from build123d import *

# Parameters (mm, degrees)
FILLET1_R             = 0.2
HEX_START             = -1.9
HEX_2_DEPTH           = 1.9
THDSCHPAT_COUNT       = 10
THDSCHPAT_PITCH       = 0.73
BODY_MOVE_COPY1_ANGLE = 90


with BuildPart() as part:
    # BodySke → BaseBody (revolve)
    with BuildSketch(Plane.XY, mode=Mode.PRIVATE) as basebody_sk:
        Polygon((0, 0), (0, 4.875), (0.725, 4.875), (3.1, 2.5), (11.555, 2.5), (12, 2.055), (12, 0), align=None)
    revolve(basebody_sk.sketch.rotate(Axis((0, 0, 0), (1, 0, 0)), 90), axis=Axis((0, 0, 0), (1, 0, 0)))

    # Fillet1
    fillet1_edges = [part.edges().sort_by_distance(p)[0] for p in [
        (3.1, 0, -2.5),
    ]]
    fillet(fillet1_edges, radius=FILLET1_R)

    # Hex 2: read off the stored shape, not the designer's step
    # Hex 2 outline → Hex 2 (cut)
    with BuildSketch(Plane.ZY.offset(HEX_START)):
        Polygon((-1.5, -0.866025404), (0, -1.732050808), (1.5, -0.866025404), (1.5, 0.866025404), (0, 1.732050808), (-1.5, 0.866025404), align=None)
    extrude(amount=HEX_2_DEPTH, mode=Mode.SUBTRACT)

    # Hex 2 2 outline → Hex 2 2 (revolve, cut)
    with BuildSketch(Plane.YX):
        Polygon((1.5, 1.9), (0, 2.766025404), (0, 1.9), align=None)
    revolve(axis=Axis((0, 0, 0), (1, 0, 0)), mode=Mode.SUBTRACT)

    # ThdSchSke → ThreadSchematic (revolve, cut)
    with BuildSketch(Plane.XY, mode=Mode.PRIVATE) as threadschematic_sk:
        Polygon((4.700001, -2.055), (4.388408645, -2.5), (4.388408645, -3.125), (5.011593355, -3.125), (5.011593355, -2.5), align=None)
    threadschematic = revolve(threadschematic_sk.sketch.rotate(Axis((-3.175, 0, 0), (1, 0, 0)), 270), axis=Axis((-3.175, 0, 0), (1, 0, 0)), mode=Mode.SUBTRACT)

    # ThdSchPat: ThreadSchematic ×10
    with Locations(*[(i * THDSCHPAT_PITCH, 0, 0) for i in range(1, THDSCHPAT_COUNT)]):
        add(threadschematic, mode=Mode.SUBTRACT)


with BuildPart() as part_1:
    # Body-Move/Copy1: moved
    add(part.part.rotate(Axis((6, 0, 0), (0, 0, -1)), BODY_MOVE_COPY1_ANGLE))


solid = part_1.part
Source: CAD feature listing. Evaluate the final solid. Frame: model axes, mm. Coordinates: 2 decimals unless noted, no trailing zeros. Loops run counter-clockwise (first coordinate to the right, second up) from the corner with the lowest first, then second, coordinate; pieces in that order, holes last. Notation, with made-up numbers: (48, -32) -> (72, -32) arc R24 cw to (72, 7) -> close; hole circle Ø4 at (-39.5, 30.5). An arc over 180 degrees is marked (long way). Answer in a Markdown table with one row per item. Add a question column.
Q1. Section A-A on y = 2.25. Return the cut outline in (x, z).
Q2. Section B-B on z = -2.25. Give the number of separate pieces and of enclosed holes in the cut face, and give its area (3 significant figures).
Q3. Ray query, line 1 along Z through (x, y) = (6.25, 5.25); line 2 along Y through (x, z) = (2, -2); line 3 along X through (y, z) = (4.5, -0.25). Return the intervals inside material, ascending.
Q4. Contact query for flat-ended pins moving along their axis: pin 1 Ø2 at (x, y) = (9, 0.5) entering from +Z; pin 2 Ø2 at (x, y) = (9, 0) entering from -Z; pin 3 Ø0.5 at (x, y) = (6.5, 5) entering from -Z. Output: stop coordinate, or through.
Computed values:
| question | item | result |
|---|---|---|
| 1 | outline | circle Ø5 at (6, 0) |
| 2 | separate pieces | 11 |
| 2 | enclosed holes | 0 |
| 2 | area | 30.1 mm^2 |
| 3 | line 1 | z = -4.84 to -1.5, 1.5 to 4.84 |
| 3 | line 2 | y = 4.87 to 6 |
| 3 | line 3 | x = 1.91 to 4.41, 7.59 to 10.09 |
| 4 | pin 1 | stops at z = 1.46 |
| 4 | pin 2 | stops at z = -1.48 |
| 4 | pin 3 | stops at z = -4.83 |
